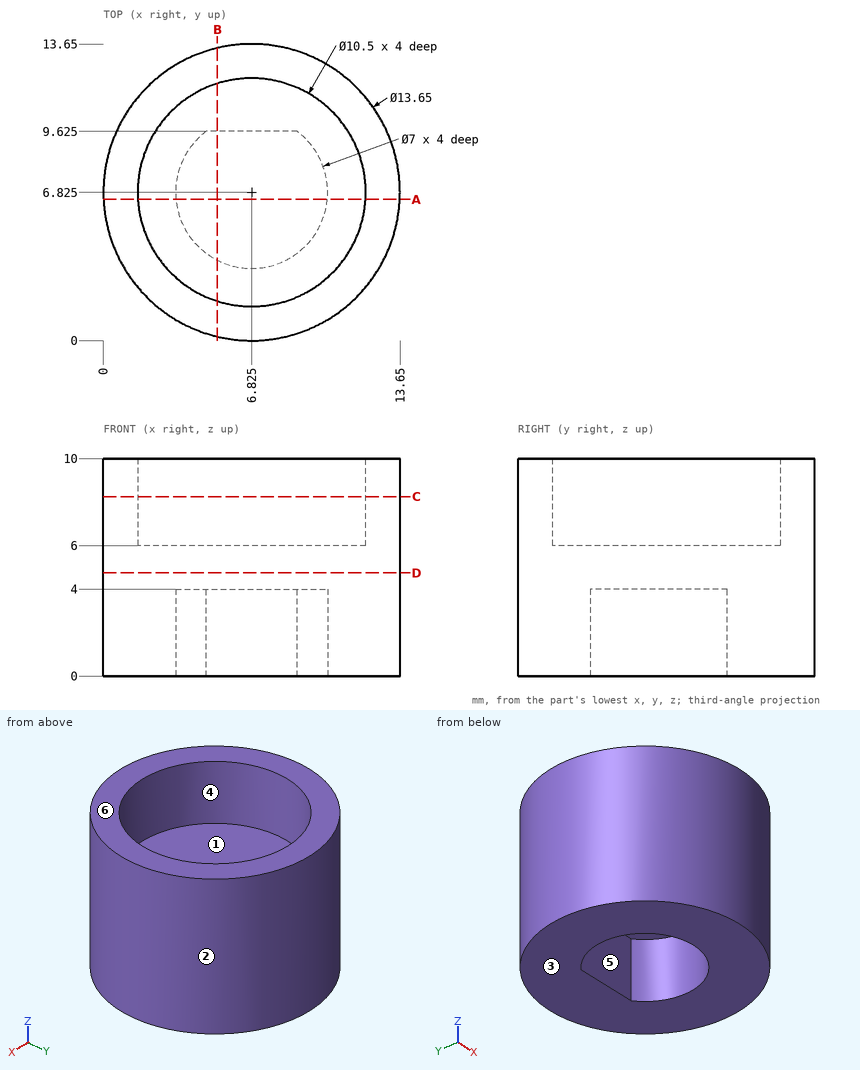
Verification items for this drawing (mm, ordinates from the low corner). A direction names the side the tool comes from. Coordinates: 2 decimals unless noted, no trailing zeros. Order: outer loops, then holes, each group sorted by start corner. A loop starts at its lowest first (then second) coordinate and runs counter-clockwise, first axis right, second up. Notation, with made-up numbers: M 1,7.5 L 26,7.5 A11 ccw 26,13.5 Z; hole C -13.5,17.25 d5. An arc over 180 degrees is marked long. Answer as a JSON object with one key per item and string values.
Q1. Release check for a two-part mould opening along X. For the marked faces 1, 2 and 3 record: released by +X, released by -X, zero draft, split by the parting line, or undercut.
Results are:
{"face 1": "undercut", "face 2": "split by the parting line", "face 3": "zero draft"}
Q2. Cross-section at B-B on x = 5.25. Record the cut outline in (y, z) (3 decimals), and give its area (3 significant figures).
Results are:
{"outline": "M 0.184,0 L 3.699,0 L 3.699,4 L 9.625,4 L 9.625,0 L 13.466,0 L 13.466,10 L 11.833,10 L 11.833,6 L 1.817,6 L 1.817,10 L 0.184,10 Z", "area": "69.0 mm²"}
Q3. Depth check by flat-ended pin: pin 1 Ø1.5 at (y, z) = (5.5, 3) entering from -X; pin 2 Ø6.5 at (x, y) = (6.825, 6.825) entering from +Z; pin 3 Ø1 at (y, z) = (2.5, 6.5) entering from -X. Enter the tip coordinate at first touch or a pass-through.
Results are:
{"pin 1": "stops at x = 0.02", "pin 2": "stops at z = 6", "pin 3": "stops at x = 1.17"}
Q4. Cross-section at C-C on z = 8.25. Record the cut outline in (x, y) (3 decimals).
Results are:
{"outline": "C 6.825,6.825 d13.65; hole C 6.825,6.825 d10.5"}
Q5. Cross-section at D-D on z = 4.75. Record the cut outline in (x, y) (3 decimals).
Results are:
{"outline": "C 6.825,6.825 d13.65"}
Q6. Cross-section at A-A on y = 6.5. Record the cut outline in (x, z), and give its area (3 significant figures).
Results are:
{"outline": "M 0.01,0 L 3.34,0 L 3.34,4 L 10.31,4 L 10.31,0 L 13.64,0 L 13.64,10 L 12.06,10 L 12.06,6 L 1.59,6 L 1.59,10 L 0.01,10 Z", "area": "66.5 mm²"}
Q7. Tool access check on the marked faces 4, 5 and 6. Record the directions out of +Z, -Z, +X, -X, +Y, -Y that give a thin tool (end or side, any length) a straight path to the whole face; none if there is none.
Results are:
{"face 4": "+Z", "face 5": "-Z", "face 6": "+Z, +X, -X, +Y, -Y"}
Q8. Scan lines: line 1 (Z direction, x = 8.75, y = 4); line 2 (Y direction, x = 4.25, z = 2.25); line 3 (X direction, y = 6.25, z = 6.5). Record each from-to range of solid material in increasing order.
Results are:
{"line 1": "z = 4 to 6", "line 2": "y = 0.5 to 4.45, 9.2 to 13.15", "line 3": "x = 0.02 to 1.61, 12.04 to 13.63"}
